from build123d import *

# Parameters (mm, degrees)
F0_R      = 4
F1_DEPTH  = 10
F2_R      = 12.5
F3_DEPTH  = 25
F9_D      = 3.5
F9_DEPTH  = 13.5
F9_TIP    = 1.0515060833
F10_DEPTH = 5


# Not quite as in the source:
# - a fillet or chamfer that OpenCascade refuses, or shapes differently, is made with other operations: its cross-section is extruded or revolved along the edge and cut away or added


with BuildPart() as f1:
    # F0 (on Top) → F1 (new body)
    with BuildSketch(Plane.XY):
        Circle(F0_R)
    extrude(amount=F1_DEPTH)

    # F2 (on face) → F3 (join)
    with BuildSketch(Plane.XY.offset(10)):
        Circle(F2_R)
    extrude(amount=F3_DEPTH)

    # F4: fillet of radius 12.499 on 2 edges, made by hand

    # F4_s1 → F4_t2 (revolve, cut)
    with BuildSketch(Plane.XZ):
        with BuildLine():
            ThreePointArc((12.5, 22.501), (8.8391276581, 31.3391276581), (0.001, 35))
            Line((0.001, 35), (12.5, 35))
            Line((12.5, 35), (12.5, 22.501))
        make_face()
    revolve(axis=Axis((0, 0, 35), (0, 0, 1)), mode=Mode.SUBTRACT)

    # F4_s3 → F4_t4 (revolve, cut)
    with BuildSketch(Plane.XZ):
        with BuildLine():
            ThreePointArc((12.5, 21.84200152), (10.1550263443, 14.5536032049), (4, 10))
            Line((4, 10), (12.5, 10))
            Line((12.5, 10), (12.5, 21.84200152))
        make_face()
    revolve(axis=Axis((0, 0, 10), (0, 0, 1)), mode=Mode.SUBTRACT)

    # F5 (on Right) → F6 (revolve, cut)
    with BuildSketch(Plane.YZ):
        with BuildLine():
            Line((12.5007824972, 23.6938826144), (10.963675566, 23.7266744822))
            ThreePointArc((10.963675566, 23.7266744822), (9.463675566, 22.2266744822), (10.963675566, 20.7266744822))
            Line((10.963675566, 20.7266744822), (12.5007824972, 20.6938826144))
            Line((12.5007824972, 20.6938826144), (12.5007824972, 23.6938826144))
        make_face()
    revolve(axis=Axis((0, 0, 10), (0, 0, -1)), mode=Mode.SUBTRACT)

    # F9
    with Locations(Plane(origin=(0, 0, 0), x_dir=(1, 0, 0), z_dir=(0, 0, -1))):
        with Locations((0, 0)):
            Hole(F9_D / 2, depth=F9_DEPTH)
            with Locations((0, 0, -(F9_DEPTH + F9_TIP / 2))):  # 118° drill point
                Cone(0, F9_D / 2, F9_TIP, mode=Mode.SUBTRACT)

    # F7 (on face) → F10 (cut)
    with BuildSketch(Plane(origin=(0, 0, 0), x_dir=(1, 0, 0), z_dir=(0, 0, -1))):
        with BuildLine():
            ThreePointArc((-2.7013885318, -2.95), (0, -4), (2.7013885318, -2.95))
            Line((2.7013885318, -2.95), (-2.7013885318, -2.95))
        make_face()
        with BuildLine():
            Line((-2.7013885318, 2.95), (2.7013885318, 2.95))
            ThreePointArc((2.7013885318, 2.95), (0, 4), (-2.7013885318, 2.95))
        make_face()
    extrude(amount=-F10_DEPTH, mode=Mode.SUBTRACT)


solid = f1.part
Could you check a few things on this model? Use its own coordinates, in mm. A direction names the side the tool comes from. Round coordinates to 2 decimals unless told otherwise and drop trailing zeros. Order: outer loops, then holes, each group sorted by start corner. A loop starts at its lowest first (then second) coordinate and runs counter-clockwise, first axis right, second up.
Q1. Imagine slicing it at A-A, the plane z = 9. List the corners of the cut face in (x, y) for me.
Geometry says:
outline: circle Ø8 at (0, 0); hole circle Ø3.5 at (0, 0)
Q2. I'm going to push flat-ended pins straight in: P1, Ø12, axis at y = 7, z = 6.5, coming from the +X side; P2, Ø1.5, axis at x = -2, y = 3.5, coming from the +Z side; P3, Ø2, axis at x = 0, y = 0, coming from the -Z side. Where does each tip first touch, or does it pass through?
Geometry says:
P1: stops at x = 6.18
P2: stops at z = 34.56
P3: stops at z = 13.95
Q3. Please list where these lines run through material, in increasing order: probe 1 along Y at (x, z) = (0, 8.5); probe 2 along Y at (x, z) = (0, 3.5); probe 3 along X at (y, z) = (1.25, 9.5).
Geometry says:
probe 1: y = -4 to -1.75, 1.75 to 4
probe 2: y = -2.95 to -1.75, 1.75 to 2.95
probe 3: x = -3.8 to -1.22, 1.22 to 3.8
Q4. Thinking about a two-plate mould opening in Y: for faces 1 (the face through (-4, 0, 6)), 2 (the face through (0, -2.95, 2)), 3 (the face through (-0.066, 0.297, 14.369)), which applies, released by +Y, released by -Y, zero draft, split by the parting line, or undercut?
Geometry says:
face 1: split by the parting line
face 2: released by -Y
face 3: undercut
Q5. Which directions (+Z, -Z, +X, -X, +Y, -Y) give clear straight access to the entire face, cutting with the end or side of a thin tool? Please do faces 4 (the face through (0, 2.95, 2)), 5 (the face through (-2, 0, 0)), 6 (the face through (-1.617, 0.67, 6.844)), 7 (the face through (0, -3.4, 5)).
Geometry says:
face 4: -Z, +X, -X, +Y
face 5: -Z, +X, -X, +Y, -Y
face 6: -Z
face 7: -Z, +X, -X, -Y
